from build123d import *

# Parameters (mm, degrees)
SKETCH1_W           = 130
SKETCH1_H           = 130
BOSS_EXTRUDE1_DEPTH = 25
SKETCH2_R           = 20.15
CUT_EXTRUDE1_DEPTH  = 12
SKETCH3_R           = 8.5
CUT_EXTRUDE2_DEPTH  = 22
SKETCH5_R           = 2.5
CUT_EXTRUDE4_DEPTH  = 30
CUT_EXTRUDE7_DEPTH  = 3


with BuildPart() as part:
    # Sketch1 → Boss-Extrude1 (new body)
    with BuildSketch(Plane(origin=(0, 0, 0), x_dir=(1, 0, 0), z_dir=(0, 1, 0))):
        Rectangle(SKETCH1_W, SKETCH1_H)
    extrude(amount=BOSS_EXTRUDE1_DEPTH)

    # Sketch2 → Cut-Extrude1 (cut)
    with BuildSketch(Plane(origin=(0, 25, 0), x_dir=(1, 0, 0), z_dir=(0, 1, 0))):
        with Locations(Location((0, 0, 0), (0, 0, 270))):
            Circle(SKETCH2_R)
    extrude(amount=-CUT_EXTRUDE1_DEPTH, mode=Mode.SUBTRACT)

    # Sketch3 → Cut-Extrude2 (cut)
    with BuildSketch(Plane(origin=(0, 13, 0), x_dir=(1, 0, 0), z_dir=(0, 1, 0))):
        with Locations(Location((0, 0, 0), (0, 0, 270))):
            Circle(SKETCH3_R)
    extrude(amount=-CUT_EXTRUDE2_DEPTH, mode=Mode.SUBTRACT)

    # Sketch5 → Cut-Extrude4 (cut)
    with BuildSketch(Plane(origin=(0, 0, 0), x_dir=(-1, 0, 0), z_dir=(0, -1, 0))):
        with Locations(Location((-22.49, -23.94, 0), (0, 0, 90))):
            Circle(SKETCH5_R)
        with Locations(Location((33.509979516, -23.987898085, 0), (0, 0, 90))):
            Circle(SKETCH5_R)
        with Locations(Location((33.07, 22.06, 0), (0, 0, 90))):
            Circle(SKETCH5_R)
        with Locations(Location((-22.92999996, 22.057895604, 0), (0, 0, 90))):
            Circle(SKETCH5_R)
    extrude(amount=-CUT_EXTRUDE4_DEPTH, mode=Mode.SUBTRACT)

    # Sketch7 → Cut-Extrude7 (cut)
    with BuildSketch(Plane(origin=(0, 25, 0), x_dir=(1, 0, 0), z_dir=(0, 1, 0))):
        Polygon((23.984601443, -20.814913357), (20.530896299, -21.08309386), (19.036294857, -24.208180504), (20.995398557, -27.065086643), (24.449103701, -26.79690614), (25.943705143, -23.671819496), align=None)
        Polygon((-32.626257702, -20.638415176), (-35.968855897, -21.54783109), (-36.852577711, -24.897313998), (-34.39370133, -27.337380993), (-31.051103134, -26.42796508), (-30.16738132, -23.078482171), align=None)
        Polygon((-34.147910167, 18.767871559), (-30.757888221, 19.480438192), (-29.679978054, 22.772566633), (-31.992089833, 25.352128441), (-35.382111779, 24.639561808), (-36.460021946, 21.347433367), align=None)
        Polygon((24.779410064, 19.128786138), (26.391388221, 22.194977003), (24.541978117, 25.12408647), (21.080589856, 24.987005071), (19.4686117, 21.920814206), (21.318021804, 18.991704739), align=None)
    extrude(amount=-CUT_EXTRUDE7_DEPTH, mode=Mode.SUBTRACT)


solid = part.part
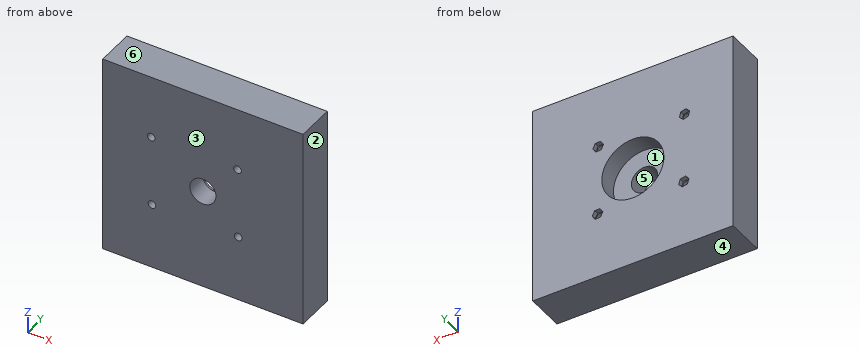
Model file for the job. Use its own axes, mm. Face numbers are marked on the shaded views. A direction names the side the tool comes from. Coordinates: 2 decimals unless noted, no trailing zeros. Loops run counter-clockwise (first coordinate to the right, second up) from the corner with the lowest first, then second, coordinate; pieces in that order, holes last. Notation, with made-up numbers: (55.25, 4) -> (110.25, 4) arc R23 ccw to (110.25, 12) -> close; hole circle Ø1 at (-34, 10.5). An arc over 180 degrees is marked (long way). Use one line per item in the form item = value. Start each with the question number.
(1) Tool access for the marked faces 1 and 2: list every direction of +Z, -Z, +X, -X, +Y, -Y with a clear straight run to the whole face (end or side of a thin tool).
(2) Flat gauge pins, fed straight in: pin 1 (2 mm diameter, centred on x = -33, z = 22.5, fed in from +Y); pin 2 (1.5 mm diameter, centred on x = 7, z = 5, fed in from +Y). Where does each tip first touch, or does it go through?
(3) Cut at D-D on x = 15. Give the cut face in (y, z).
(4) Probe probe 1 along X at (y, z) = (11.25, 23.94); probe 2 along Z at (x, y) = (-33.5, 15.25); probe 3 along Z at (x, y) = (22.93, 6.5). List the from-to ranges inside material, lowest first. Write a range as from..to.
(5) Cut at A-A on z = 0. Give the cut face in (x, y), and give its area (3 significant figures).
(6) Cut at C-C on y = 18. Give the cut face in (x, z), and give its area (3 significant figures).
(7) Cut at B-B on x = 0. Give the cut face in (y, z), and give its area (3 significant figures).
(8) Pull direction Z, two halves, no side cores. Call the marked faces 3, 4, 5 and 6: pulls with the +Z half, pulls with the -Z half, needs draft (parallel to the pull), parting line crosses it, or undercut.
Values:
q1.face_1 = +Y
q1.face_2 = +Z, -Z, +X, +Y, -Y
q2.pin_1 = 22
q2.pin_2 = 13
q3.outline = (0, -65) -> (25, -65) -> (25, -13.45) -> (13, -13.45) -> (13, 13.45) -> (25, 13.45) -> (25, 65) -> (0, 65) -> close
q4.probe_1 = -65..-36.01, -31.01..19.99, 24.99..65
q4.probe_2 = -65..-24.52, -19.6..21.49, 26.49..65
q4.probe_3 = -65..-24.56, -19.56..21.48, 26.4..65
q5.outline = (-65, 0) -> (-8.5, 0) -> (-8.5, 13) -> (-20.15, 13) -> (-20.15, 25) -> (-65, 25) -> close; (8.5, 0) -> (65, 0) -> (65, 25) -> (20.15, 25) -> (20.15, 13) -> (8.5, 13) -> close
q5.area = 2,550 mm2
q6.outline = (-65, -65) -> (65, -65) -> (65, 65) -> (-65, 65) -> close; hole circle Ø5 at (-33.51, 23.99); hole circle Ø5 at (-33.07, -22.06); hole circle Ø40.3 at (0, 0); hole circle Ø5 at (22.49, 23.94); hole circle Ø5 at (22.93, -22.06)
q6.area = 15,500 mm2
q7.outline = (0, -65) -> (25, -65) -> (25, -20.15) -> (13, -20.15) -> (13, -8.5) -> (0, -8.5) -> close; (0, 8.5) -> (13, 8.5) -> (13, 20.15) -> (25, 20.15) -> (25, 65) -> (0, 65) -> close
q7.area = 2,550 mm2
q8.face_3 = needs draft
q8.face_4 = pulls with the -Z half
q8.face_5 = undercut
q8.face_6 = pulls with the +Z half
